Part model, mm, in its own coordinate system. Face numbers are marked on the shaded views. Round coordinates to 2 decimals unless told otherwise and drop trailing zeros. Order: outer loops, then holes, each group sorted by start corner. A loop starts at its lowest first (then second) coordinate and runs counter-clockwise, first axis right, second up. Notation, with made-up numbers: M 63.25,60.5 L 79.25,60.5 A17 cw 79.25,69.5 Z; hole C 43,76 d3. An arc over 180 degrees is marked long. Write each question's results on one line, items separated by ' | '. Start each with the question number.
1. Probe L1, parallel to Z at x = 0, y = 19.25; L2, parallel to Y at x = -4, z = -45.5; L3, parallel to Z at x = -19.5, y = 8.5. List the from-to ranges inside material, lowest first. Write a range as [from, to].
2. Two-plate mould, pull along X, no slides. Class the marked faces 1, 2, 3 and 4: +X half, -X half, draft (parallel to the pull), parting line (faces both ways), or undercut.
3. Band-saw the part on C-C, the plane z = -18. List the corners of the cut face in (x, y), then the cut area to 3 significant figures.
4. Band-saw the part on D-D, the plane x = -13. List the corners of the cut face in (y, z).
5. Band-saw the part on B-B, the plane x = -2. List the corners of the cut face in (y, z).
6. Band-saw the part on A-A, the plane y = 19.5. List the corners of the cut face in (x, z).
7. Drop flat-ended pins along their axis: pin 1 Ø4 at (x, y) = (-24, 17) entering from +Z; pin 2 Ø3 at (y, z) = (11.5, 35) entering from +X; pin 3 Ø10 at (y, z) = (17, -39) entering from +X; pin 4 Ø11 at (y, z) = (13, -45.26) entering from +X. Give the stop position or say it passes through.
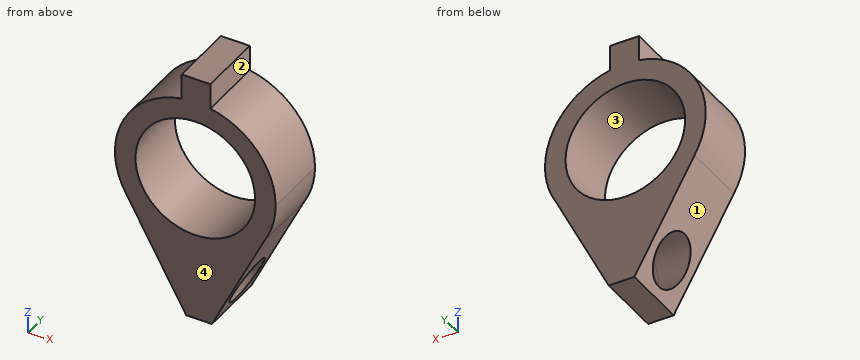
```python
from build123d import *

# Parameters (mm, degrees)
F0_R     = 23.3
F2_DEPTH = 26
F3_D     = 18
F3_DEPTH = 31.301
F4_D     = 18
F4_DEPTH = 31.301


with BuildPart() as f2:
    # F0 (on Front) → F2 (new body)
    with BuildSketch(Plane.XZ):
        with BuildLine():
            ThreePointArc((-5.3364344982, 30.8417325526), (0.278406123, 31.2987617971), (5.8842282742, 30.7419234534))
            Line((5.8842282742, 30.7419234534), (5.8842282742, 40.749304027))
            Line((5.8842282742, 40.749304027), (-5.3364344982, 40.749304027))
            Line((-5.3364344982, 40.749304027), (-5.3364344982, 30.8417325526))
        make_face()
        with BuildLine():
            ThreePointArc((26.9505900946, -15.9171509245), (30.1930742883, -8.2503493877), (31.3, 0))
            ThreePointArc((31.3, 0), (24.1232910792, 19.9438418442), (5.8842282742, 30.7419234534))
            ThreePointArc((5.8842282742, 30.7419234534), (0.278406123, 31.2987617971), (-5.3364344982, 30.8417325526))
            ThreePointArc((-5.3364344982, 30.8417325526), (-28.4114639762, 13.1331151952), (-26.9505900946, -15.9171509245))
            ThreePointArc((-26.9505900946, -15.9171509245), (-14.8696278527, -27.5424067126), (1.4777821376, -31.2650949136))
            ThreePointArc((1.4777821376, -31.2650949136), (16.1534186201, -26.8096450347), (26.9505900946, -15.9171509245))
        make_face()
        Circle(F0_R, mode=Mode.SUBTRACT)
        with BuildLine():
            Line((6.4777821376, -57.4513469467), (26.9505900946, -15.9171509245))
            ThreePointArc((26.9505900946, -15.9171509245), (16.1534186201, -26.8096450347), (1.4777821376, -31.2650949136))
            Line((1.4777821376, -31.2650949136), (1.4777821376, -57.4513469467))
            Line((1.4777821376, -57.4513469467), (6.4777821376, -57.4513469467))
        make_face()
        with BuildLine():
            Line((1.4777821376, -57.4513469467), (1.4777821376, -31.2650949136))
            ThreePointArc((1.4777821376, -31.2650949136), (-14.8696278527, -27.5424067126), (-26.9505900946, -15.9171509245))
            Line((-26.9505900946, -15.9171509245), (-3.5222178624, -57.4513469467))
            Line((-3.5222178624, -57.4513469467), (1.4777821376, -57.4513469467))
        make_face()
    extrude(amount=-F2_DEPTH)

    # F3 (through all, one way)
    with BuildSketch(Plane.YZ):
        with Locations((13, -45.2576093376)):
            Circle(F3_D / 2)
    extrude(amount=-F3_DEPTH, mode=Mode.SUBTRACT)

    # F4 (through all, one way)
    with BuildSketch(Plane(origin=(0, 0, 0), x_dir=(0, 1, 0), z_dir=(-1, 0, 0))):
        with Locations((12.9997157162, 45.1954063838)):
            Circle(F4_D / 2)
    extrude(amount=-F4_DEPTH, mode=Mode.SUBTRACT)


solid = f2.part
```
Solution:
1) L1: [-57.45, -51.73], [-38.72, -23.3], [23.3, 40.75] | L2: [0, 4], [22, 26] | L3: [-29.13, -12.75], [12.75, 24.48]
2) face 1: -X half | face 2: +X half | face 3: undercut | face 4: draft
3) outline: M -25.78,0 L -14.79,0 L -14.79,26 L -25.78,26 Z; M 14.79,0 L 25.92,0 L 25.92,26 L 14.79,26 Z | area: 575 mm^2
4) outline: M 0,-40.65 L 5.27,-40.65 A9 cw 20.73,-40.65 L 26,-40.65 L 26,-19.34 L 0,-19.34 Z; M 0,19.34 L 26,19.34 L 26,28.47 L 0,28.47 Z
5) outline: M 0,-57.45 L 26,-57.45 L 26,-23.21 L 0,-23.21 Z; M 0,23.21 L 26,23.21 L 26,40.75 L 0,40.75 Z; hole C 13,-45.26 d18
6) outline: M -26.95,-15.92 L -13.91,-39.03 L 0,-39.03 L 0,-38.97 L 15.59,-38.97 L 26.95,-15.92 A31.3 ccw 5.88,30.74 L 5.88,40.75 L -5.34,40.75 L -5.34,30.84 A31.3 ccw Z; M -6.89,-51.48 L -3.52,-57.45 L 6.48,-57.45 L 9.45,-51.42 L 0,-51.42 L 0,-51.48 Z; hole C 0,0 d46.6
7) pin 1: z = 22.26 | pin 2: x = 5.88 | pin 3: x = 18.04 | pin 4: through
